Can you work these out from the model? Positions are in its coordinate system, mm. Face numbers are marked on the shaded views. Round coordinates to 2 decimals unless told otherwise and drop trailing zeros. Loops run counter-clockwise (first coordinate to the right, second up) from the corner with the lowest first, then second, coordinate; pieces in that order, holes last. Notation, with made-up numbers: M 24,46.25 L 33,46.25 A17 ccw 33,68.25 Z; hole C 38,7 d10. An arc over 180 degrees is marked long. Use a Markdown table: item, result. Add a question column.
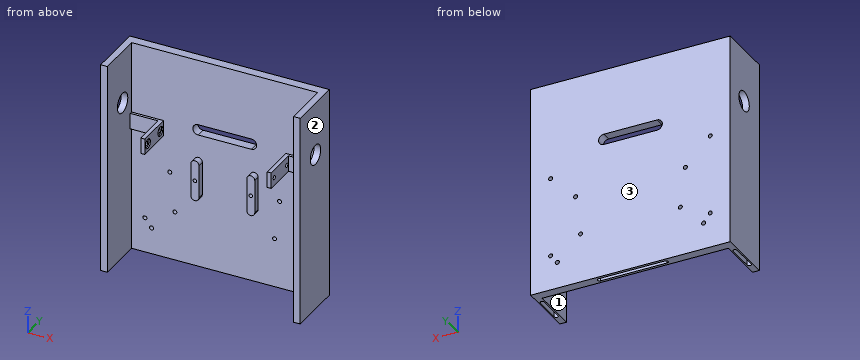
```python
from build123d import *

# Parameters (mm, degrees)
BOSS_EXTRUDE1_DEPTH = 160
CUT_EXTRUDE1_DEPTH  = 32
SKETCH3_R           = 7.5
CUT_EXTRUDE2_DEPTH  = 210
SKETCH5_R           = 1.5
CUT_EXTRUDE4_DEPTH  = 210
CUT_EXTRUDE6_DEPTH  = 20
SKETCH8_R           = 1.55
CUT_EXTRUDE7_DEPTH  = 10
SKETCH9_W           = 24
SKETCH9_H           = 12
BOSS_EXTRUDE3_DEPTH = 2
SKETCH10_W          = 3
SKETCH10_H          = 12
BOSS_EXTRUDE4_DEPTH = 25
SKETCH11_R          = 3.5
CUT_EXTRUDE8_DEPTH  = 1
SKETCH12_R          = 1.55
CUT_EXTRUDE9_DEPTH  = 3
SKETCH13_R          = 1.5
SKETCH13_R_2        = 1.55
CUT_EXTRUDE10_DEPTH = 10
SKETCH14_R          = 1.375
BOSS_EXTRUDE5_DEPTH = 5


with BuildPart() as part:
    # Sketch1 → Boss-Extrude1 (new body)
    with BuildSketch(Plane.XY):
        Polygon((-95.061728395, -14.551440329), (-95.061728395, 27.448559671), (54.938271605, 27.448559671), (54.938271605, -14.551440329), (49.938271605, -14.551440329), (49.938271605, 20.448559671), (-90.061728395, 20.448559671), (-90.061728395, -14.551440329), align=None)
    extrude(amount=BOSS_EXTRUDE1_DEPTH)

    # Sketch2 → Cut-Extrude1 (cut)
    with BuildSketch(Plane(origin=(0, 0, 0), x_dir=(-1, 0, 0), z_dir=(0, 0, -1))):
        with BuildLine():
            Line((-50.938271605, 15.448559671), (-50.938271605, -4.551440329))
            ThreePointArc((-50.938271605, -4.551440329), (-52.438271605, -6.051440329), (-53.938271605, -4.551440329))
            Line((-53.938271605, -4.551440329), (-53.938271605, 15.448559671))
            ThreePointArc((-53.938271605, 15.448559671), (-52.438271605, 16.948559671), (-50.938271605, 15.448559671))
        make_face()
        with BuildLine():
            Line((-4.938271605, 25.448559671), (45.061728395, 25.448559671))
            ThreePointArc((45.061728395, 25.448559671), (46.561728395, 23.948559671), (45.061728395, 22.448559671))
            Line((45.061728395, 22.448559671), (-4.938271605, 22.448559671))
            ThreePointArc((-4.938271605, 22.448559671), (-6.438271605, 23.948559671), (-4.938271605, 25.448559671))
        make_face()
        with BuildLine():
            Line((94.061728395, 15.448559671), (94.061728395, -4.551440329))
            ThreePointArc((94.061728395, -4.551440329), (92.561728395, -6.051440329), (91.061728395, -4.551440329))
            Line((91.061728395, -4.551440329), (91.061728395, 15.448559671))
            ThreePointArc((91.061728395, 15.448559671), (92.561728395, 16.948559671), (94.061728395, 15.448559671))
        make_face()
    extrude(amount=-CUT_EXTRUDE1_DEPTH, mode=Mode.SUBTRACT)

    # Sketch3 → Cut-Extrude2 (cut)
    with BuildSketch(Plane.ZY.offset(95.061728395)):
        with Locations((120, 7.448559671)):
            Circle(SKETCH3_R)
    extrude(amount=-CUT_EXTRUDE2_DEPTH, mode=Mode.SUBTRACT)

    # Sketch5 → Cut-Extrude4 (cut)
    with BuildSketch(Plane(origin=(0, 27.448559671, 0), x_dir=(1, 0, 0), z_dir=(0, 1, 0))):
        with Locations(Location((-80.061728395, -26.5, 0), (0, 0, 180))):
            Circle(SKETCH5_R)
        with Locations(Location((39.938271605, -26.5, 0), (0, 0, 180))):
            Circle(SKETCH5_R)
        with Locations(Location((-80.061728395, -86.5, 0), (0, 0, 180))):
            Circle(SKETCH5_R)
        with Locations(Location((39.938271605, -86.5, 0), (0, 0, 180))):
            Circle(SKETCH5_R)
    extrude(amount=-CUT_EXTRUDE4_DEPTH, mode=Mode.SUBTRACT)

    # Sketch7 → Cut-Extrude6 (cut)
    with BuildSketch(Plane(origin=(0, 27.448559671, 0), x_dir=(1, 0, 0), z_dir=(0, 1, 0))):
        with BuildLine():
            Line((-40.061728395, -102), (-0.061728395, -102))
            ThreePointArc((-0.061728395, -102), (3.938271605, -106), (-0.061728395, -110))
            Line((-0.061728395, -110), (-40.061728395, -110))
            ThreePointArc((-40.061728395, -110), (-44.061728395, -106), (-40.061728395, -102))
        make_face()
    extrude(amount=-CUT_EXTRUDE6_DEPTH, mode=Mode.SUBTRACT)

    # Sketch8 → Cut-Extrude7 (cut)
    with BuildSketch(Plane(origin=(0, 27.448559671, 0), x_dir=(1, 0, 0), z_dir=(0, 1, 0))):
        with Locations(Location((-75.061728395, -20, 0), (0, 0, 180))):
            Circle(SKETCH8_R)
        with Locations(Location((34.938271605, -20, 0), (0, 0, 180))):
            Circle(SKETCH8_R)
    extrude(amount=-CUT_EXTRUDE7_DEPTH, mode=Mode.SUBTRACT)

    # Sketch9 → Boss-Extrude3 (add)
    with BuildSketch(Plane.XZ.offset(-20.448559671)):
        with Locations((37.938271605, 100)):
            Rectangle(SKETCH9_W, SKETCH9_H)
    boss_extrude3 = extrude(amount=BOSS_EXTRUDE3_DEPTH)

    # Sketch10 → Boss-Extrude4 (add)
    with BuildSketch(Plane.XZ.offset(-18.448559671)):
        with Locations((27.438271605, 100)):
            Rectangle(SKETCH10_W, SKETCH10_H)
    boss_extrude4 = extrude(amount=BOSS_EXTRUDE4_DEPTH)

    # Sketch11 → Cut-Extrude8 (cut)
    with BuildSketch(Plane.ZY.offset(-25.938271605)):
        with Locations(Location((100, 15.948559671, 0), (0, 0, 270))):
            Circle(SKETCH11_R)
        with Locations(Location((100, -2.051440329, 0), (0, 0, 270))):
            Circle(SKETCH11_R)
    cut_extrude8 = extrude(amount=-CUT_EXTRUDE8_DEPTH, mode=Mode.SUBTRACT)

    # Sketch12 → Cut-Extrude9 (cut)
    with BuildSketch(Plane.ZY.offset(-26.938271605)):
        with Locations(Location((100, 15.948559671, 0), (0, 0, 270))):
            Circle(SKETCH12_R)
        with Locations(Location((100, -2.051440329, 0), (0, 0, 270))):
            Circle(SKETCH12_R)
    cut_extrude9 = extrude(amount=-CUT_EXTRUDE9_DEPTH, mode=Mode.SUBTRACT)

    # Mirror1: Boss-Extrude3, Boss-Extrude4, Cut-Extrude8, Cut-Extrude9 across plane
    add(boss_extrude3.mirror(Plane.ZY.offset(20.061728395)))
    add(boss_extrude4.mirror(Plane.ZY.offset(20.061728395)))
    add(cut_extrude8.mirror(Plane.ZY.offset(20.061728395)), mode=Mode.SUBTRACT)
    add(cut_extrude9.mirror(Plane.ZY.offset(20.061728395)), mode=Mode.SUBTRACT)

    # Sketch13 → Cut-Extrude10 (cut)
    with BuildSketch(Plane(origin=(0, 27.448559671, 0), x_dir=(1, 0, 0), z_dir=(0, 1, 0))):
        with Locations(Location((17.438271605, -37.265826534, 0), (0, 0, 180))):
            Circle(SKETCH13_R)
        with Locations(Location((-57.561728395, -37.265826534, 0), (0, 0, 180))):
            Circle(SKETCH13_R)
        with Locations(Location((-61.341728395, -67.223803809, 0), (0, 0, 180))):
            Circle(SKETCH13_R)
        with Locations(Location((21.218271605, -67.223803809, 0), (0, 0, 180))):
            Circle(SKETCH13_R_2)
    extrude(amount=-CUT_EXTRUDE10_DEPTH, mode=Mode.SUBTRACT)

    # Sketch14 → Boss-Extrude5 (add)
    # profile 1 of 2: a face of its own
    with BuildSketch(Plane.XZ.offset(-20.448559671)):
        with BuildLine():
            Line((5.139369782, 81.650400065), (5.139369782, 56.650400065))
            ThreePointArc((5.139369782, 56.650400065), (2.139369782, 53.650400065), (-0.860630218, 56.650400065))
            Line((-0.860630218, 56.650400065), (-0.860630218, 81.650400065))
            ThreePointArc((-0.860630218, 81.650400065), (2.139369782, 84.650400065), (5.139369782, 81.650400065))
        make_face()
        with Locations((2.139369782, 69.150400065)):
            Circle(SKETCH14_R, mode=Mode.SUBTRACT)
    # profile 2 of 2: a face of its own
    with BuildSketch(Plane.XZ.offset(-20.448559671)):
        with BuildLine():
            Line((-36.860630218, 81.650400065), (-36.860630218, 56.650400065))
            ThreePointArc((-36.860630218, 56.650400065), (-39.860630218, 53.650400065), (-42.860630218, 56.650400065))
            Line((-42.860630218, 56.650400065), (-42.860630218, 81.650400065))
            ThreePointArc((-42.860630218, 81.650400065), (-39.860630218, 84.650400065), (-36.860630218, 81.650400065))
        make_face()
        with Locations((-39.860630218, 69.150400065)):
            Circle(SKETCH14_R, mode=Mode.SUBTRACT)
    extrude(amount=BOSS_EXTRUDE5_DEPTH)


solid = part.part
```
(1) Thinking about a two-plate mould opening in X: for the marked faces 1, 2 and 3, which applies, released by +X, released by -X, zero draft, split by the parting line, or undercut?
(2) Suppose I cut it at B-B on z = 120. List the corners of the cut face in (x, y) for me, and give its area (3 significant figures).
(3) Suppose I cut it at A-A on x = -35. List the corners of the cut face in (y, z) for me, and give its area (3 significant figures).
(4) If I drill on probe 1 along X at (y, z) = (8, 71); probe 2 along X at (y, z) = (23.5, 27); probe 3 along X at (y, z) = (25, 20.5), over which ranges is the centre line in solid material (lowest first)? Write a range as [from, to].
(5) I'm going to push flat-ended pins straight in: pin 1 (3 mm diameter, centred on x = -11.5, z = 109.5, fed in from -Y); pin 2 (13.5 mm diameter, centred on y = 7.45, z = 120, fed in from -X); pin 3 (3.5 mm diameter, centred on x = -67.5, z = 98.5, fed in from -Y); pin 4 (2 mm diameter, centred on x = 3, z = 69.5, fed in from -Y). Where does each tip first touch, or does it pass through?
(6) Suppose I cut it at D-D on x = -53.5. List the corners of the cut face in (y, z) for me.
(7) Suppose I cut it at C-C on z = 43.5. List the corners of the cut face in (x, y) for me.
Results below:
| question | item | result |
|---|---|---|
| 1 | face 1 | undercut |
| 1 | face 2 | released by +X |
| 1 | face 3 | zero draft |
| 2 | outline | M -95.06,-14.55 L -90.06,-14.55 L -90.06,-0.05 L -95.06,-0.05 Z; M -95.06,14.95 L -90.06,14.95 L -90.06,20.45 L 49.94,20.45 L 49.94,14.95 L 54.94,14.95 L 54.94,27.45 L -95.06,27.45 Z; M 49.94,-14.55 L 54.94,-14.55 L 54.94,-0.05 L 49.94,-0.05 Z |
| 2 | area | 1,250 mm² |
| 3 | outline | M 20.45,0 L 22.45,0 L 22.45,32 L 25.45,32 L 25.45,0 L 27.45,0 L 27.45,102 L 20.45,102 Z; M 20.45,110 L 27.45,110 L 27.45,160 L 20.45,160 Z |
| 3 | area | 968 mm² |
| 4 | probe 1 | x = [-95.06, -90.06], [49.94, 54.94] |
| 4 | probe 2 | x = [-95.06, -81.48], [-78.65, -46.49], [6.37, 38.52], [41.35, 54.94] |
| 4 | probe 3 | x = [-95.06, -76.53], [-73.59, -46.13], [6.01, 33.47], [36.41, 54.94] |
| 5 | pin 1 | stops at y = 20.45 |
| 5 | pin 2 | passes through |
| 5 | pin 3 | stops at y = -6.55 |
| 5 | pin 4 | stops at y = 15.45 |
| 6 | outline | M 20.45,0 L 27.45,0 L 27.45,160 L 20.45,160 Z |
| 7 | outline | M -95.06,-14.55 L -90.06,-14.55 L -90.06,20.45 L 49.94,20.45 L 49.94,-14.55 L 54.94,-14.55 L 54.94,27.45 L -95.06,27.45 Z |
